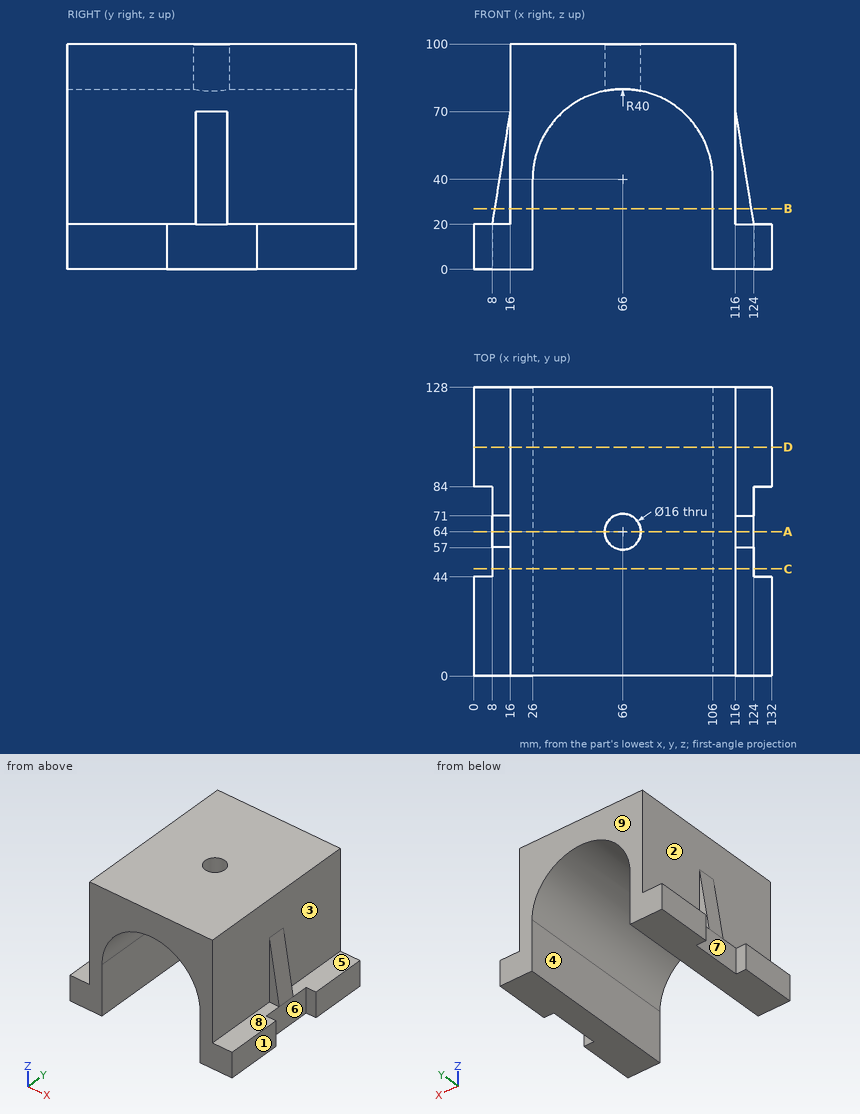
Study the drawing (mm; zero at the part's minimum x, y, z) and answer. A direction names the side the tool comes from. Give positions to 0.01 mm unless a question says otherwise; leave off trailing zeros. Loops run counter-clockwise (first coordinate to the right, second up) from the corner with the lowest first, then second, coordinate; pieces in that order, holes last. Notation, with made-up numbers: (-34.5, 38) -> (-11.5, 38) arc R18 cw to (-11.5, 56) -> close; hole circle Ø11 at (77.25, 70). An arc over 180 degrees is marked (long way). Use a Markdown table: item, result. Add a question column.
1) The part is cut by section B-B, the plane z = 27. Determine the outline of the cut face in (x, y).
2) The part is cut by section C-C, the plane y = 47.5. Determine the outline of the cut face in (x, z).
3) The part is cut by section D-D, the plane y = 101.5. Determine the outline of the cut face in (x, z), plus the area to 3 significant figures.
4) The part is cut by section A-A, the plane y = 64. Determine the outline of the cut face in (x, z), plus the area to 3 significant figures.
5) For a pull along Y with two mould halves and no side action, classify the marked faces 6, 7, 8 and 9 as +Y half, -Y half, draft (parallel to the pull), parting line (faces both ways), or undercut.
6) Each of these flat-tipped pins is pushed along its axis until it touches: P1, Ø6.5, axis at x = 12, z = 38, coming from the -Y side; P2, Ø8, axis at x = 6.5, y = 95.5, coming from the +Z side; P3, Ø1, axis at y = 85.5, z = 58, coming from the +X side. Where does it stop, or does it pass through?
7) Consider line 1 along Y through (x, z) = (66, 95); line 2 along X through (y, z) = (105, 26.5); line 3 along X through (y, z) = (95.5, 13). Determine where each line is inside the solid, lowest interval first.
8) Which of the six approach directions +Z, -Z, +X, -X, +Y, -Y give full straight-line access (tool end or side, diameter ignored) to the marked faces 1, 2, 3, 4 and 5?
Reported:
| question | item | result |
|---|---|---|
| 1 | outline | (9.12, 57) -> (16, 57) -> (16, 0) -> (26, 0) -> (26, 128) -> (16, 128) -> (16, 71) -> (9.12, 71) -> close; (106, 0) -> (116, 0) -> (116, 57) -> (122.88, 57) -> (122.88, 71) -> (116, 71) -> (116, 128) -> (106, 128) -> close |
| 2 | outline | (8, 0) -> (26, 0) -> (26, 40) arc R40 cw to (106, 40) -> (106, 0) -> (124, 0) -> (124, 20) -> (116, 20) -> (116, 100) -> (16, 100) -> (16, 20) -> (8, 20) -> close |
| 3 | outline | (0, 0) -> (26, 0) -> (26, 40) arc R40 cw to (106, 40) -> (106, 0) -> (132, 0) -> (132, 20) -> (116, 20) -> (116, 100) -> (16, 100) -> (16, 20) -> (0, 20) -> close |
| 3 | area | 4,930 mm^2 |
| 4 | outline | (8, 0) -> (26, 0) -> (26, 40) arc R40 cw to (58, 79.19) -> (58, 100) -> (16, 100) -> (16, 70) -> (8, 20) -> close; (74, 79.19) arc R40 cw to (106, 40) -> (106, 0) -> (124, 0) -> (124, 20) -> (116, 70) -> (116, 100) -> (74, 100) -> close |
| 4 | area | 4,680 mm^2 |
| 5 | face 6 | undercut |
| 5 | face 7 | undercut |
| 5 | face 8 | draft |
| 5 | face 9 | +Y half |
| 6 | P1 | stops at y = 57 |
| 6 | P2 | stops at z = 20 |
| 6 | P3 | stops at x = 116 |
| 7 | line 1 | y = 0 to 56, 72 to 128 |
| 7 | line 2 | x = 16 to 26, 106 to 116 |
| 7 | line 3 | x = 0 to 26, 106 to 132 |
| 8 | face 1 | +Z, -Z, +X, +Y, -Y |
| 8 | face 2 | +Z, -X |
| 8 | face 3 | +Z, +X |
| 8 | face 4 | -Z, +Y, -Y |
| 8 | face 5 | +Z, +X, +Y |
